```python
from build123d import *

# Parameters (mm, degrees)
F0_W      = 8.9408
F0_H      = 5.461
F1_DEPTH  = 111.76
F2_T      = -2.54
F4_DEPTH  = 25.4
F5_DEPTH  = 25.4
F7_DEPTH  = 25.4
F8_W      = 2.5400399546
F8_H      = 7.62
F9_DEPTH  = 5.08
F10_W     = 2.5400002226
F10_H     = 15.24
F10_H_2   = 7.62
F11_DEPTH = 5.08
F12_W     = 6.223
F12_H     = 6.223
F13_DEPTH = 25.4


with BuildPart() as f1:
    # F0 (on Top) → F1 (new body)
    with BuildSketch(Plane.XY):
        with BuildLine():
            Line((54.9210952491, 19.4422315109), (-8.5789047509, 19.4422315109))
            ThreePointArc((-8.5789047509, 19.4422315109), (-17.8451170094, 11.099606562), (-21.2789029923, -0.8866853785))
            Line((-21.2789029923, -0.8866853785), (9.0740952491, -0.8866853785))
            Line((9.0740952491, -0.8866853785), (34.4740952491, -0.8866853785))
            Line((34.4740952491, -0.8866853785), (34.4740952491, 4.5743146215))
            Line((34.4740952491, 4.5743146215), (43.4148952491, 4.5743146215))
            Line((43.4148952491, 4.5743146215), (43.4148952491, -0.8866853785))
            Line((43.4148952491, -0.8866853785), (67.6266683049, -0.8866853785))
            ThreePointArc((67.6266683049, -0.8866853785), (64.1599500532, 11.0815657388), (54.9210952491, 19.4422315109))
        make_face()
        with Locations((38.9444952491, 1.8438146215)):
            Rectangle(F0_W, F0_H)
    extrude(amount=-F1_DEPTH)

    # F2
    f2_openings = [f1.faces().sort_by_distance(p)[0] for p in [
        (23.173883, -0.886685, -55.88),
    ]]
    offset(amount=F2_T, openings=f2_openings)

    # F3 (on face) → F4 (cut)
    with BuildSketch(Plane.XY):
        Polygon((1.3137662318, 1.1936101676), (1.3137662318, -0.8866853785), (9.0607662318, -0.8866853785), (9.0607662318, 1.1936101676), (1.3270952491, 1.1936101676), align=None)
    extrude(amount=-F4_DEPTH, mode=Mode.SUBTRACT)

    # F0 (on Top) → F5 (cut)
    with BuildSketch(Plane.XY):
        with Locations((38.9444952491, 1.8438146215)):
            Rectangle(F0_W, F0_H)
    extrude(amount=-F5_DEPTH, mode=Mode.SUBTRACT)

    # F6 (on face) → F7 (cut)
    with BuildSketch(Plane(origin=(0, 0, -111.76), x_dir=(1, 0, 0), z_dir=(0, 0, -1))):
        with BuildLine():
            Line((29.0158826563, 0.8866853785), (17.3318826563, 0.8866853785))
            ThreePointArc((17.3318826563, 0.8866853785), (23.1738826563, -4.9553146215), (29.0158826563, 0.8866853785))
        make_face()
    extrude(amount=-F7_DEPTH, mode=Mode.SUBTRACT)

    # F8 (on face) → F9 (join)
    with BuildSketch(Plane.XZ.offset(0.8866853785)):
        with Locations((66.3566483276, -31.75)):
            Rectangle(F8_W, F8_H)
        with Locations((66.3566483276, -39.37)):
            Rectangle(F8_W, F8_H)
        with Locations((66.3566483276, -80.01)):
            Rectangle(F8_W, F8_H)
        with Locations((66.3566483276, -87.63)):
            Rectangle(F8_W, F8_H)
    extrude(amount=F9_DEPTH)

    # F10 (on face) → F11 (join)
    with BuildSketch(Plane.XZ.offset(0.8866853785)):
        with Locations((-20.008902881, -35.56)):
            Rectangle(F10_W, F10_H)
        with Locations((-20.008902881, -80.01)):
            Rectangle(F10_W, F10_H_2)
        with Locations((-20.008902881, -87.63)):
            Rectangle(F10_W, F10_H_2)
    extrude(amount=F11_DEPTH)

    # F12 (on face) → F13 (cut)
    with BuildSketch(Plane(origin=(0, 19.4422315109, 0), x_dir=(-1, 0, 0), z_dir=(0, 1, 0))):
        with Locations((-4.1845952491, -24.8285)):
            Rectangle(F12_W, F12_H)
        with Locations((-10.4075952491, -24.8285)):
            Rectangle(F12_W, F12_H)
        with Locations((-10.4075952491, -31.0515)):
            Rectangle(F12_W, F12_H)
        with Locations((-4.1845952491, -31.0515)):
            Rectangle(F12_W, F12_H)
        with Locations((-35.9345952491, -24.8285)):
            Rectangle(F12_W, F12_H)
        with Locations((-42.1575952491, -24.8285)):
            Rectangle(F12_W, F12_H)
        with Locations((-42.1575952491, -31.0515)):
            Rectangle(F12_W, F12_H)
        with Locations((-35.9345952491, -31.0515)):
            Rectangle(F12_W, F12_H)
        with BuildLine():
            Line((-39.0460952491, -83.82), (-39.0460952491, -79.375))
            ThreePointArc((-39.0460952491, -79.375), (-42.1891848914, -80.6769103576), (-43.4910952491, -83.82))
            Line((-43.4910952491, -83.82), (-39.0460952491, -83.82))
        make_face()
        with BuildLine():
            Line((-39.0460952491, -88.265), (-39.0460952491, -83.82))
            Line((-39.0460952491, -83.82), (-43.4910952491, -83.82))
            ThreePointArc((-43.4910952491, -83.82), (-42.1891848914, -86.9630896424), (-39.0460952491, -88.265))
        make_face()
        with BuildLine():
            ThreePointArc((-39.0460952491, -88.265), (-35.9030056067, -86.9630896424), (-34.6010952491, -83.82))
            Line((-34.6010952491, -83.82), (-39.0460952491, -83.82))
            Line((-39.0460952491, -83.82), (-39.0460952491, -88.265))
        make_face()
        with BuildLine():
            Line((-39.0460952491, -83.82), (-34.6010952491, -83.82))
            ThreePointArc((-34.6010952491, -83.82), (-35.9030056067, -80.6769103576), (-39.0460952491, -79.375))
            Line((-39.0460952491, -79.375), (-39.0460952491, -83.82))
        make_face()
        with BuildLine():
            ThreePointArc((-7.2960952491, -79.375), (-10.4391848914, -80.6769103576), (-11.7410952491, -83.82))
            Line((-11.7410952491, -83.82), (-7.2960952491, -83.82))
            Line((-7.2960952491, -83.82), (-7.2960952491, -79.375))
        make_face()
        with BuildLine():
            Line((-7.2960952491, -83.82), (-11.7410952491, -83.82))
            ThreePointArc((-11.7410952491, -83.82), (-10.4391848914, -86.9630896424), (-7.2960952491, -88.265))
            Line((-7.2960952491, -88.265), (-7.2960952491, -83.82))
        make_face()
        with BuildLine():
            Line((-2.8510952491, -83.82), (-7.2960952491, -83.82))
            Line((-7.2960952491, -83.82), (-7.2960952491, -88.265))
            ThreePointArc((-7.2960952491, -88.265), (-4.1530056067, -86.9630896424), (-2.8510952491, -83.82))
        make_face()
        with BuildLine():
            ThreePointArc((-2.8510952491, -83.82), (-4.1530056067, -80.6769103576), (-7.2960952491, -79.375))
            Line((-7.2960952491, -79.375), (-7.2960952491, -83.82))
            Line((-7.2960952491, -83.82), (-2.8510952491, -83.82))
        make_face()
    extrude(amount=-F13_DEPTH, mode=Mode.SUBTRACT)


solid = f1.part
```
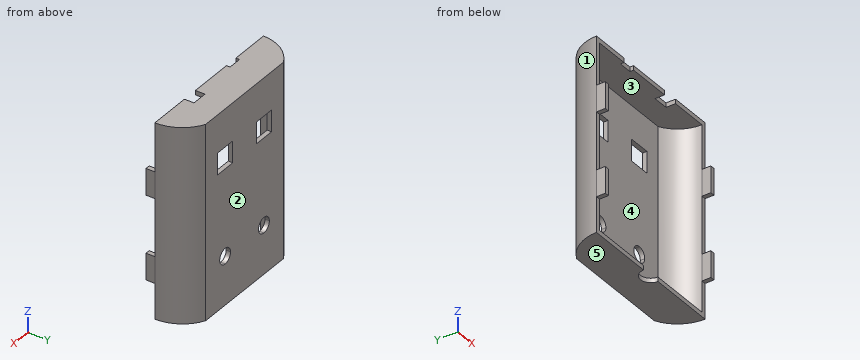
Work out the finished part from the listing and answer in its coordinate system (mm). Face numbers are marked on the shaded views. A direction names the side the tool comes from. Coordinates: 2 decimals unless noted, no trailing zeros. Write each loop counter-clockwise with the first axis right and the second up, starting at its lowest first coordinate (ties: lowest second). Pieces come first, ordered by that corner, then holes.
Q1. A cutting plane is placed at C-C, the plane x = 53. Give the vertices of the cut face in (y, z).
Q2. Which of the six approach directions +Z, -Z, +X, -X, +Y, -Y give full straight-line access (tool end or side, diameter ignored) to the marked faces 4 and 5?
Q3. Determine the mould class of the marked faces 1, 2 and 3 for opening direction X: released by +X, released by -X, zero draft, split by the parting line, or undercut.
Q4. A cutting plane is placed at D-D, the plane x = 5. Give the vertices of the cut face in (y, z), then the cut area to 3 significant figures.
Q5. Each of these flat-tipped pins is pushed along its axis until it touches: pin 1 Ø3 at (x, z) = (39.5, -1.5) entering from -Y; pin 2 Ø2 at (y, z) = (11, -74) entering from -X; pin 3 Ø2 at (x, z) = (39.5, -61.5) entering from -Y. Where does it stop, or does it pass through?
Q6. A cutting plane is placed at A-A, the plane y = -3.5. Give the vertices of the cut face in (x, z).
Q7. A cutting plane is placed at B-B, the plane z = -45. Give the vertices of the cut face in (x, y), then the cut area to 3 significant figures.
Q8. Find the intervals of material crossed by line 1 (Z direction, x = -2.5, y = 15.5); line 2 (X direction, y = 8.5, z = -98.5); line 3 (X direction, y = 2, z = -76), in increasing order.
Findings below:
1. outline: (-0.89, -111.76) - (19.44, -111.76) - (19.44, 0) - (-0.89, 0) - (-0.89, -2.54) - (16.9, -2.54) - (16.9, -109.22) - (-0.89, -109.22) - close
2. face 4: -Y
2. face 5: -Z, +X, -X, +Y, -Y
3. face 1: released by -X
3. face 2: zero draft
3. face 3: undercut
4. outline: (-0.89, -111.76) - (19.44, -111.76) - (19.44, -87.63) - (16.9, -87.63) - (16.9, -109.22) - (-0.89, -109.22) - close; (1.19, -2.54) - (16.9, -2.54) - (16.9, -21.72) - (19.44, -21.72) - (19.44, 0) - (1.19, 0) - close; (16.9, -80.01) - (19.44, -80.01) - (19.44, -34.16) - (16.9, -34.16) - close
4. area: 318 mm2
5. pin 1: stops at y = 4.57
5. pin 2: stops at x = -18.49
5. pin 3: stops at y = 16.9
6. outline: (-21.28, -91.44) - (-18.74, -91.44) - (-18.74, -76.2) - (-21.28, -76.2) - close; (-21.28, -43.18) - (-18.74, -43.18) - (-18.74, -27.94) - (-21.28, -27.94) - close; (65.09, -91.44) - (67.63, -91.44) - (67.63, -76.2) - (65.09, -76.2) - close; (65.09, -43.18) - (67.63, -43.18) - (67.63, -27.94) - (65.09, -27.94) - close
7. outline: (-21.28, -0.89) - (-18.74, -0.89) arc R20.07 cw to (-7.97, 16.9) - (54.31, 16.9) arc R20.27 cw to (65.09, -0.89) - (67.63, -0.89) arc R22.81 ccw to (54.92, 19.44) - (-8.58, 19.44) arc R22.61 ccw to start
7. area: 279 mm2
8. line 1: z = -111.76 to -109.22, -2.54 to 0
8. line 2: x = -19.24 to -16.41, 62.72 to 65.55
8. line 3: x = -21.09 to -18.53, 64.86 to 67.43
